Verification items for the finished model (mm, model axes). Face numbers are marked on the shaded views. A direction names the side the tool comes from. Round coordinates to 2 decimals unless told otherwise and drop trailing zeros. Loops run counter-clockwise (first coordinate to the right, second up) from the corner with the lowest first, then second, coordinate; pieces in that order, holes last. Notation, with made-up numbers: M 30,33.25 L 77,33.25 A17 ccw 77,59.25 Z; hole C 54.25,78.5 d4. An arc over 180 degrees is marked long. One line per item, written item: value.
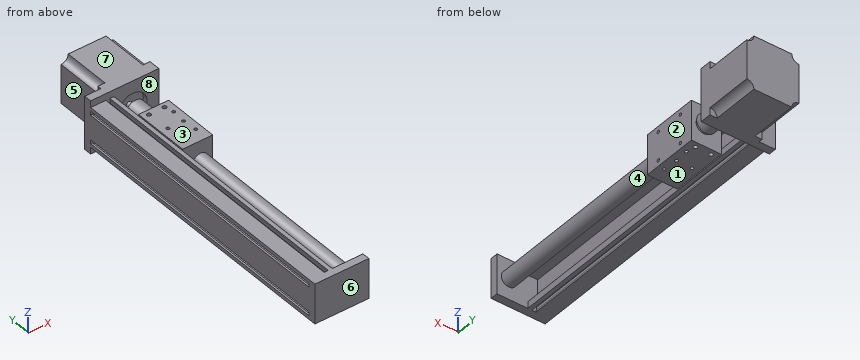
from build123d import *

# Parameters (mm, degrees)
SKETCH1_W                      = 57
SKETCH1_H                      = 42
BOSS_EXTRUDE1_DEPTH            = 8
BOSS_EXTRUDE2_DEPTH            = 297
SKETCH3_W                      = 72
SKETCH3_H                      = 56
BOSS_EXTRUDE3_DEPTH            = 8
SKETCH4_W                      = 55
SKETCH4_H                      = 56
BOSS_EXTRUDE4_DEPTH            = 54
CUT_EXTRUDE1_DEPTH             = 50
SKETCH6_R                      = 8
BOSS_EXTRUDE5_DEPTH            = 268.3
SKETCH7_W                      = 31.8
SKETCH7_H                      = 42
BOSS_EXTRUDE6_DEPTH            = 30
SKETCH8_R                      = 10
BOSS_EXTRUDE7_DEPTH            = 25
SKETCH9_R                      = 15
CUT_EXTRUDE2_DEPTH             = 5
BOSS_EXTRUDE8_REACH            = 67.7
SKETCH10_R                     = 3.175
SKETCH11_W                     = 4.3
SKETCH11_H                     = 297
CUT_EXTRUDE3_DEPTH             = 5.4
SKETCH12_W                     = 3.6
SKETCH12_H                     = 297
CUT_EXTRUDE4_DEPTH             = 2.7
SKETCH13_W                     = 4.3
SKETCH13_H                     = 297
CUT_EXTRUDE5_DEPTH             = 6.8
SKETCH14_W                     = 3.3
SKETCH14_H                     = 297
CUT_EXTRUDE6_DEPTH             = 3.4
M4X0_7_TAPPED_HOLE1_D          = 3.3
M4X0_7_TAPPED_HOLE1_DEPTH      = 10.1
M4X0_7_TAPPED_HOLE1_TIP        = 0.991420021
M4X0_7_TAPPED_HOLE2_AT_2_COUNT = 2
M4X0_7_TAPPED_HOLE2_AT_2_PITCH = 30
M4X0_7_TAPPED_HOLE2_AT_3_COUNT = 2
M4X0_7_TAPPED_HOLE2_AT_3_PITCH = 15.044018745
M4X0_7_TAPPED_HOLE2_AT_4_COUNT = 2
M4X0_7_TAPPED_HOLE2_AT_4_PITCH = 23.162955338
M5X0_8_TAPPED_HOLE1_AT_2_COUNT = 2
M5X0_8_TAPPED_HOLE1_AT_2_PITCH = 16.5


with BuildPart() as part:
    # Sketch1 → Boss-Extrude1 (new body)
    with BuildSketch(Plane(origin=(0, 0, 0), x_dir=(1, 0, 0), z_dir=(0, 1, 0))):
        with Locations((28.5, 0)):
            Rectangle(SKETCH1_W, SKETCH1_H)
    extrude(amount=BOSS_EXTRUDE1_DEPTH)

    # Sketch2 → Boss-Extrude2 (add)
    with BuildSketch(Plane(origin=(0, 8, 0), x_dir=(1, 0, 0), z_dir=(0, 1, 0))):
        Polygon((0, 21), (0, -21), (24.5, -21), (24.5, -14), (14.1, -14), (14.1, 14), (24.5, 14), (24.5, 21), align=None)
    extrude(amount=BOSS_EXTRUDE2_DEPTH)

    # Sketch3 → Boss-Extrude3 (add)
    with BuildSketch(Plane(origin=(0, 305, 0), x_dir=(1, 0, 0), z_dir=(0, 1, 0))):
        with Locations((36, 0)):
            Rectangle(SKETCH3_W, SKETCH3_H)
    extrude(amount=BOSS_EXTRUDE3_DEPTH)

    # Sketch4 → Boss-Extrude4 (add)
    with BuildSketch(Plane(origin=(0, 313, 0), x_dir=(1, 0, 0), z_dir=(0, 1, 0))):
        with Locations((44.5, 0)):
            Rectangle(SKETCH4_W, SKETCH4_H)
    extrude(amount=BOSS_EXTRUDE4_DEPTH)

    # Sketch5 → Cut-Extrude1 (cut)
    with BuildSketch(Plane(origin=(0, 367, 0), x_dir=(1, 0, 0), z_dir=(0, 1, 0))):
        with BuildLine():
            Line((17, 28), (17, 20.5))
            ThreePointArc((17, 20.5), (22.303300859, 22.696699141), (24.5, 28))
            Line((24.5, 28), (17, 28))
        make_face()
        with BuildLine():
            Line((72, 28), (64.5, 28))
            ThreePointArc((64.5, 28), (66.696699141, 22.696699141), (72, 20.5))
            Line((72, 20.5), (72, 28))
        make_face()
        with BuildLine():
            Line((72, -28), (72, -20.5))
            ThreePointArc((72, -20.5), (66.696699141, -22.696699141), (64.5, -28))
            Line((64.5, -28), (72, -28))
        make_face()
        with BuildLine():
            Line((17, -28), (24.5, -28))
            ThreePointArc((24.5, -28), (22.303300859, -22.696699141), (17, -20.5))
            Line((17, -20.5), (17, -28))
        make_face()
    extrude(amount=-CUT_EXTRUDE1_DEPTH, mode=Mode.SUBTRACT)

    # Sketch6 → Boss-Extrude5 (add)
    with BuildSketch(Plane(origin=(0, 8, 0), x_dir=(1, 0, 0), z_dir=(0, 1, 0))):
        with Locations((44.5, 0)):
            Circle(SKETCH6_R)
    extrude(amount=BOSS_EXTRUDE5_DEPTH)

    # Sketch7 → Boss-Extrude6 (add, symmetric)
    with BuildSketch(Plane(origin=(0, 243, 0), x_dir=(1, 0, 0), z_dir=(0, 1, 0))):
        with Locations((41.6, 0)):
            Rectangle(SKETCH7_W, SKETCH7_H)
    extrude(amount=BOSS_EXTRUDE6_DEPTH, both=True)

    # Sketch8 → Boss-Extrude7 (add)
    with BuildSketch(Plane(origin=(0, 276.3, 0), x_dir=(1, 0, 0), z_dir=(0, 1, 0))):
        with Locations((44.5, 0)):
            Circle(SKETCH8_R)
    extrude(amount=BOSS_EXTRUDE7_DEPTH)

    # Sketch9 → Cut-Extrude2 (cut)
    with BuildSketch(Plane.XZ.offset(-305)):
        with Locations((44.5, 0)):
            Circle(SKETCH9_R)
    extrude(amount=-CUT_EXTRUDE2_DEPTH, mode=Mode.SUBTRACT)

    # Sketch10 → Boss-Extrude8 (add, up to next)
    with BuildSketch(Plane(origin=(0, 301.3, 0), x_dir=(1, 0, 0), z_dir=(0, 1, 0)), mode=Mode.PRIVATE) as boss_extrude8_sk1:
        with Locations((44.5, 0)):
            Circle(SKETCH10_R)
    boss_extrude8_tool1 = extrude(boss_extrude8_sk1.sketch, amount=BOSS_EXTRUDE8_REACH, mode=Mode.PRIVATE) - part.part
    add(boss_extrude8_tool1.solids().sort_by_distance((44.5, 301.3, 0))[0])

    # Sketch11 → Cut-Extrude3 (cut)
    with BuildSketch(Plane(origin=(0, 0, -21), x_dir=(-1, 0, 0), z_dir=(0, 0, -1))):
        with Locations((-18.15, 156.5)):
            Rectangle(SKETCH11_W, SKETCH11_H)
    cut_extrude3 = extrude(amount=-CUT_EXTRUDE3_DEPTH, mode=Mode.SUBTRACT)

    # Sketch12 → Cut-Extrude4 (cut, symmetric)
    with BuildSketch(Plane(origin=(18.15, 0, 0), x_dir=(0, 0, -1), z_dir=(1, 0, 0))):
        with Locations((17.4, 156.5)):
            Rectangle(SKETCH12_W, SKETCH12_H)
    cut_extrude4 = extrude(amount=CUT_EXTRUDE4_DEPTH, both=True, mode=Mode.SUBTRACT)

    # Mirror1: Cut-Extrude3, Cut-Extrude4 across plane
    add(cut_extrude3.mirror(Plane.XY), mode=Mode.SUBTRACT)
    add(cut_extrude4.mirror(Plane.XY), mode=Mode.SUBTRACT)

    # Sketch13 → Cut-Extrude5 (cut)
    with BuildSketch(Plane.ZY):
        with Locations((15, 156.5)):
            Rectangle(SKETCH13_W, SKETCH13_H)
    cut_extrude5 = extrude(amount=-CUT_EXTRUDE5_DEPTH, mode=Mode.SUBTRACT)

    # Sketch14 → Cut-Extrude6 (cut, symmetric)
    with BuildSketch(Plane.XY.offset(15)):
        with Locations((3.65, 156.5)):
            Rectangle(SKETCH14_W, SKETCH14_H)
    cut_extrude6 = extrude(amount=CUT_EXTRUDE6_DEPTH, both=True, mode=Mode.SUBTRACT)

    # Mirror2: Cut-Extrude5, Cut-Extrude6 across plane
    add(cut_extrude5.mirror(Plane.XY), mode=Mode.SUBTRACT)
    add(cut_extrude6.mirror(Plane.XY), mode=Mode.SUBTRACT)

    # M4x0.7 Tapped Hole1
    with Locations(Plane(origin=(57.5, 0, 0), x_dir=(0, 0, -1), z_dir=(1, 0, 0))):
        with Locations((-15, 258), (15, 258), (15, 228), (-15, 228)):
            Hole(M4X0_7_TAPPED_HOLE1_D / 2, depth=M4X0_7_TAPPED_HOLE1_DEPTH)
            with Locations((0, 0, -(M4X0_7_TAPPED_HOLE1_DEPTH + M4X0_7_TAPPED_HOLE1_TIP / 2))):  # 118° drill point
                Cone(0, M4X0_7_TAPPED_HOLE1_D / 2, M4X0_7_TAPPED_HOLE1_TIP, mode=Mode.SUBTRACT)

    # Sketch23 → M4x0.7 Tapped Hole2 (revolve, cut)
    with BuildSketch(Plane(origin=(51.15, 228, 21), x_dir=(0, -1, 0), z_dir=(1, 0, 0))):
        Polygon((0, 0), (0, 6.991420021), (1.65, 6), (1.65, 0), align=None)
    m4x0_7_tapped_hole2 = revolve(axis=Axis((51.15, 228, 27.35), (0, 0, -1)), mode=Mode.SUBTRACT)

    # M4x0.7 Tapped Hole2 at 2: M4x0.7 Tapped Hole2 ×2
    with Locations(*[(0, i * M4X0_7_TAPPED_HOLE2_AT_2_PITCH, 0) for i in range(1, M4X0_7_TAPPED_HOLE2_AT_2_COUNT)]):
        add(m4x0_7_tapped_hole2, mode=Mode.SUBTRACT)

    # M4x0.7 Tapped Hole2 at 3: M4x0.7 Tapped Hole2 ×2
    with Locations(*[Vector(-0.07644234, 0.997074004, 0) * (i * M4X0_7_TAPPED_HOLE2_AT_3_PITCH) for i in range(1, M4X0_7_TAPPED_HOLE2_AT_3_COUNT)]):
        add(m4x0_7_tapped_hole2, mode=Mode.SUBTRACT)

    # M4x0.7 Tapped Hole2 at 4: M4x0.7 Tapped Hole2 ×2
    with Locations(*[Vector(-0.761992576, 0.647585758, 0) * (i * M4X0_7_TAPPED_HOLE2_AT_4_PITCH) for i in range(1, M4X0_7_TAPPED_HOLE2_AT_4_COUNT)]):
        add(m4x0_7_tapped_hole2, mode=Mode.SUBTRACT)

    # Sketch25 → M5x0.8 Tapped Hole1 (revolve, cut)
    with BuildSketch(Plane(origin=(32.5, 267.5, 21), x_dir=(0, -1, 0), z_dir=(1, 0, 0))):
        Polygon((0, 0), (0, 11.2618073), (2.1, 10), (2.1, 0), align=None)
    m5x0_8_tapped_hole1 = revolve(axis=Axis((32.5, 267.5, 27.35), (0, 0, -1)), mode=Mode.SUBTRACT)

    # M5x0.8 Tapped Hole1 at 2: M5x0.8 Tapped Hole1 ×2
    with Locations(*[(i * M5X0_8_TAPPED_HOLE1_AT_2_PITCH, 0, 0) for i in range(1, M5X0_8_TAPPED_HOLE1_AT_2_COUNT)]):
        add(m5x0_8_tapped_hole1, mode=Mode.SUBTRACT)

    # Mirror3: M5x0.8 Tapped Hole1, M4x0.7 Tapped Hole2 across plane
    add(m5x0_8_tapped_hole1.mirror(Plane.XY), mode=Mode.SUBTRACT)
    add(m4x0_7_tapped_hole2.mirror(Plane.XY), mode=Mode.SUBTRACT)

    # Mirror3 copy 1 sketch → Mirror3 copy 1 (revolve, cut)
    with BuildSketch(Plane(origin=(49, 267.5, -21), x_dir=(0, -1, 0), z_dir=(1, 0, 0))):
        Polygon((0, 0), (0, -11.2618073), (2.1, -10), (2.1, 0), align=None)
    revolve(axis=Axis((49, 267.5, -27.35), (0, 0, -1)), mode=Mode.SUBTRACT)

    # Mirror3 copy 2 sketch → Mirror3 copy 2 (revolve, cut)
    with BuildSketch(Plane(origin=(51.15, 258, -21), x_dir=(0, -1, 0), z_dir=(1, 0, 0))):
        Polygon((0, 0), (0, -6.991420021), (1.65, -6), (1.65, 0), align=None)
    revolve(axis=Axis((51.15, 258, -27.35), (0, 0, -1)), mode=Mode.SUBTRACT)

    # Mirror3 copy 3 sketch → Mirror3 copy 3 (revolve, cut)
    with BuildSketch(Plane(origin=(50, 243, -21), x_dir=(0, -1, 0), z_dir=(1, 0, 0))):
        Polygon((0, 0), (0, -6.991420021), (1.65, -6), (1.65, 0), align=None)
    revolve(axis=Axis((50, 243, -27.35), (0, 0, -1)), mode=Mode.SUBTRACT)

    # Mirror3 copy 4 sketch → Mirror3 copy 4 (revolve, cut)
    with BuildSketch(Plane(origin=(33.5, 243, -21), x_dir=(0, -1, 0), z_dir=(1, 0, 0))):
        Polygon((0, 0), (0, -6.991420021), (1.65, -6), (1.65, 0), align=None)
    revolve(axis=Axis((33.5, 243, -27.35), (0, 0, -1)), mode=Mode.SUBTRACT)


solid = part.part
(1) Mould release check, pull along Y, two halves, no side actions. Record for the marked faces 6, 7 and 8: +Y half, -Y half, draft (parallel to the pull), parting line (faces both ways), or undercut.
Completed:
face 6: -Y half
face 7: draft
face 8: undercut
(2) Thickness scan on L1, parallel to Z at x = 3.5, y = 165; L2, parallel to X at y = 228, z = -17.95; L3, parallel to X at y = 228, z = -17.1. Record the ranges inside material, lowest first. Write a range as from..to.
Completed:
L1: z = -21..-18.4, -11.6..11.6, 18.4..21
L2: x = 0..2, 5.3..15.45, 20.85..24.5, 25.7..49.5, 52.8..57.5
L3: x = 6.8..15.45, 20.85..24.5, 25.7..49.5, 52.8..57.5
(3) Sectioned sample at B-B on y = 324. Enter the section's corners in (x, z), and give its area (3 significant figures).
Completed:
outline: M 17,-20.5 A7.5 cw 24.5,-28 L 64.5,-28 A7.5 cw 72,-20.5 L 72,20.5 A7.5 cw 64.5,28 L 24.5,28 A7.5 cw 17,20.5 Z
area: 2,900 mm^2
(4) Depth check by flat-ended pin: pin 1 Ø4 at (y, z) = (258, -15) entering from +X; pin 2 Ø2 at (x, y) = (50, 243) entering from -Z; pin 3 Ø2 at (y, z) = (113, -20) entering from +X; pin 4 Ø6 at (y, z) = (205, -16) entering from -X. Enter the tip coordinate at first touch or a pass-through.
Completed:
pin 1: stops at x = 57.5
pin 2: stops at z = -14.61
pin 3: stops at x = 24.5
pin 4: stops at x = 0
(5) Tool access check on the marked faces 1, 2, 3, 4 and 5. Record the directions out of +Z, -Z, +X, -X, +Y, -Y that give a thin tool (end or side, any length) a straight path to the whole face; none if there is none.
Completed:
face 1: -Z, +X, -X, -Y
face 2: +Z, -Z, +X, -Y
face 3: +Z, +X, -X, -Y
face 4: none
face 5: +Z, -Z, -X, +Y
(6) Sectioned sample at C-C on x = 10. Enter the section's corners in (y, z).
Completed:
outline: M 0,-21 L 305,-21 L 305,-28 L 313,-28 L 313,28 L 305,28 L 305,21 L 0,21 Z
